CAD build for the part. Positions are in the model's coordinates, mm. Face numbers are marked on the shaded views. A direction names the side the tool comes from. Coordinates: 2 decimals unless noted, no trailing zeros. Loops run counter-clockwise (first coordinate to the right, second up) from the corner with the lowest first, then second, coordinate; pieces in that order, holes last. Notation, with made-up numbers: (89.5, -26) -> (121.5, -26) arc R23 cw to (121.5, -7) -> close; hole circle Ø2 at (18.25, 85.25). An arc over 180 degrees is marked (long way). Write each question's results on one line, items separated by ' | '.
```python
from build123d import *

# Parameters (mm, degrees)
SKETCH4_R           = 1.155
BOSS_EXTRUDE1_DEPTH = 0.75
SKETCH6_R           = 2.5
SKETCH6_R_2         = 1.155
BOSS_EXTRUDE2_DEPTH = 3.25


with BuildPart() as part:
    # Sketch4 → Boss-Extrude1 (new body)
    with BuildSketch(Plane.XY.offset(-4.75)):
        with BuildLine():
            ThreePointArc((-2.275132275, 2.766302827), (0, 2.11510717), (2.275132275, 2.766302827))
            ThreePointArc((2.275132275, 2.766302827), (7.26, 0), (2.275132275, -2.766302827))
            ThreePointArc((2.275132275, -2.766302827), (0, -2.11510717), (-2.275132275, -2.766302827))
            ThreePointArc((-2.275132275, -2.766302827), (-7.26, 0), (-2.275132275, 2.766302827))
        make_face()
        with Locations((-4, 0)):
            Circle(SKETCH4_R, mode=Mode.SUBTRACT)
        with Locations((4, 0)):
            Circle(SKETCH4_R, mode=Mode.SUBTRACT)
    boss_extrude1 = extrude(amount=BOSS_EXTRUDE1_DEPTH)

    # Sketch6 → Boss-Extrude2 (add)
    # profile 1 of 2: a face of its own
    with BuildSketch(Plane.XY.offset(-4)):
        with Locations(Location((-4, 0, 0), (0, 0, 180))):
            Circle(SKETCH6_R)
        with Locations((-4, 0)):
            Circle(SKETCH6_R_2, mode=Mode.SUBTRACT)
    # profile 2 of 2: a face of its own
    with BuildSketch(Plane.XY.offset(-4)):
        with Locations(Location((4, 0, 0), (0, 0, 180))):
            Circle(SKETCH6_R)
        with Locations((4, 0)):
            Circle(SKETCH6_R_2, mode=Mode.SUBTRACT)
    extrude(amount=BOSS_EXTRUDE2_DEPTH)

    # Mirror1: Boss-Extrude1 across plane
    add(boss_extrude1.mirror(Plane.XY.offset(-2.75)))


solid = part.part
```
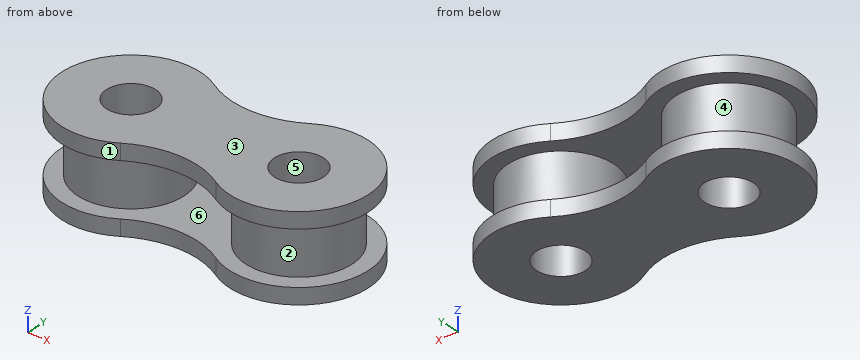
Q1. Cut at D-D on x = 5.75. Write the cut outline in (y, z).
Results are:
outline: (-2.75, -4.75) -> (2.75, -4.75) -> (2.75, -4) -> (1.79, -4) -> (1.79, -1.5) -> (2.75, -1.5) -> (2.75, -0.75) -> (-2.75, -0.75) -> (-2.75, -1.5) -> (-1.79, -1.5) -> (-1.79, -4) -> (-2.75, -4) -> close
Q2. Which spindle directions (+Z, -Z, +X, -X, +Y, -Y) get a long thin tool onto all of the face, cutting with end or side? Do the marked faces 5 and 6. Say none if no direction does.
Results are:
face 5: +Z, -Z | face 6: none
Q3. Pull direction Z, two halves, no side cores. Call the marked faces 1, 2, 3 and 4: +Z half, -Z half, draft (parallel to the pull), parting line (faces both ways), or undercut.
Results are:
face 1: draft | face 2: undercut | face 3: +Z half | face 4: undercut
Q4. Cut at A-A on y = 0. Write the cut outline in (x, z) (3 decimals).
Results are:
outline: (-7.26, -4.75) -> (-5.155, -4.75) -> (-5.155, -0.75) -> (-7.26, -0.75) -> (-7.26, -1.5) -> (-6.5, -1.5) -> (-6.5, -4) -> (-7.26, -4) -> close; (-2.845, -4.75) -> (2.845, -4.75) -> (2.845, -0.75) -> (-2.845, -0.75) -> close; (5.155, -4.75) -> (7.26, -4.75) -> (7.26, -4) -> (6.5, -4) -> (6.5, -1.5) -> (7.26, -1.5) -> (7.26, -0.75) -> (5.155, -0.75) -> close; hole (-1.5, -4) -> (1.5, -4) -> (1.5, -1.5) -> (-1.5, -1.5) -> close
Q5. Cut at B-B on x = -4. Write the cut outline in (y, z) (3 decimals).
Results are:
outline: (-3.26, -4.75) -> (-1.155, -4.75) -> (-1.155, -0.75) -> (-3.26, -0.75) -> (-3.26, -1.5) -> (-2.5, -1.5) -> (-2.5, -4) -> (-3.26, -4) -> close; (1.155, -4.75) -> (3.26, -4.75) -> (3.26, -4) -> (2.5, -4) -> (2.5, -1.5) -> (3.26, -1.5) -> (3.26, -0.75) -> (1.155, -0.75) -> close
Q6. Drop flat-ended pins along their axis: pin 1 (2 mm diameter, centred on x = -1, z = -3.5, fed in from -Y); pin 2 (1.4 mm diameter, centred on x = -4, y = 0, fed in from -Z). Give the stop position or say it passes through.
Results are:
pin 1: y = -2.54 | pin 2: through
Q7. Wall check: L1, parallel to Z at x = 3, y = -3; L2, parallel to Y at x = -4, z = -1.7 (3 decimals); L3, parallel to X at y = 0.75, z = -2.1. Give the ranges that are in metal, low to high. Write a range as from..to.
Results are:
L1: -4.75..-4, -1.5..-0.75 | L2: -2.5..-1.155, 1.155..2.5 | L3: -6.38..-4.88, -3.12..-1.62, 1.62..3.12, 4.88..6.38
Q8. Cut at C-C on z = -3.2. Write the cut outline in (x, y) (3 decimals), and give its area (3 significant figures).
Results are:
outline: circle Ø5 at (-4, 0); circle Ø5 at (4, 0); hole circle Ø2.31 at (-4, 0); hole circle Ø2.31 at (4, 0) | area: 30.9 mm^2
